Part print with two shaded views. Sizes in mm from the minimum x, y, z corner. Coordinates: 2 decimals unless noted, no trailing zeros. Loops run counter-clockwise (first coordinate to the right, second up) from the corner with the lowest first, then second, coordinate; pieces in that order, holes last.
Item 1: Drill centre lines: line 1 along Y through (x, z) = (11.43, 1.1); line 2 along X through (y, z) = (1.27, 1.6); line 3 along Y through (x, z) = (6.35, 1.45). Where is each one in solid material? Low to high.
Item 2: Cut at B-B (y = 6.35). List the corners of the cut face in (x, z).
Item 3: Cut at D-D (y = 3.81). List the corners of the cut face in (x, z).
Item 4: Mould opens along X. For the marked faces 1, 2 and 3 say: released by +X, released by -X, zero draft, split by the parting line, or undercut.
Item 5: Cut at C-C (x = 1.27). List the corners of the cut face in (y, z).
Item 6: Cut at A-A (z = 0.4). List the corners of the cut face in (x, y).
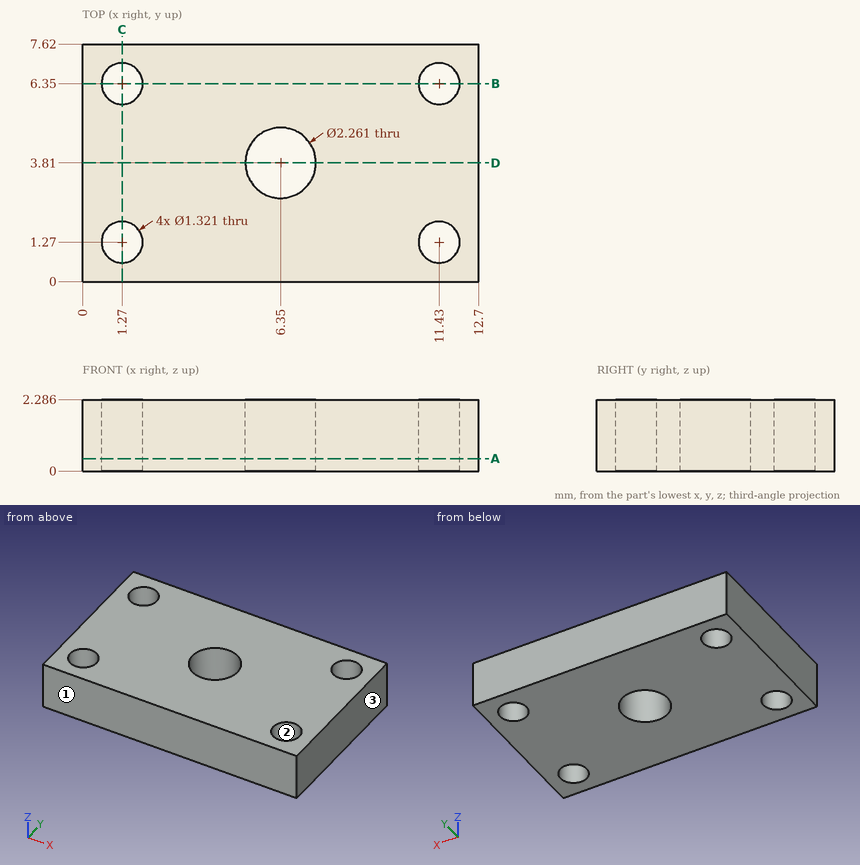
Filled sheet:
1. line 1: y = 0 to 0.61, 1.93 to 5.69, 7.01 to 7.62
1. line 2: x = 0 to 0.61, 1.93 to 10.77, 12.09 to 12.7
1. line 3: y = 0 to 2.68, 4.94 to 7.62
2. outline: (0, 0) - (0.61, 0) - (0.61, 2.29) - (0, 2.29) - close; (1.93, 0) - (10.77, 0) - (10.77, 2.29) - (1.93, 2.29) - close; (12.09, 0) - (12.7, 0) - (12.7, 2.29) - (12.09, 2.29) - close
3. outline: (0, 0) - (5.22, 0) - (5.22, 2.29) - (0, 2.29) - close; (7.48, 0) - (12.7, 0) - (12.7, 2.29) - (7.48, 2.29) - close
4. face 1: zero draft
4. face 2: undercut
4. face 3: released by +X
5. outline: (0, 0) - (0.61, 0) - (0.61, 2.29) - (0, 2.29) - close; (1.93, 0) - (5.69, 0) - (5.69, 2.29) - (1.93, 2.29) - close; (7.01, 0) - (7.62, 0) - (7.62, 2.29) - (7.01, 2.29) - close
6. outline: (0, 0) - (12.7, 0) - (12.7, 7.62) - (0, 7.62) - close; hole circle Ø1.32 at (1.27, 1.27); hole circle Ø1.32 at (1.27, 6.35); hole circle Ø2.26 at (6.35, 3.81); hole circle Ø1.32 at (11.43, 1.27); hole circle Ø1.32 at (11.43, 6.35)
